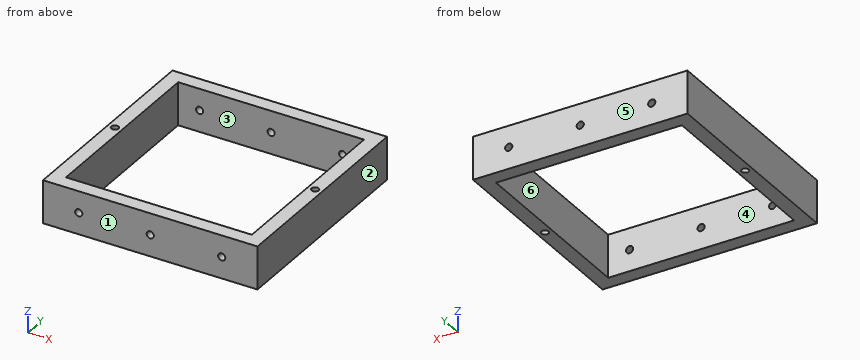
Autodesk Inventor part; units mm, degrees
ref_plane "YZ Plane" through (0, 0, 0) normal (1, 0, 0) x (0, 1, 0)
ref_plane "XZ Plane" through (0, 0, 0) normal (0, 1, 0) x (-1, 0, 0)
ref_plane "XY Plane" through (0, 0, 0) normal (0, 0, 1) x (1, 0, 0)
sketch "Boceto1" plane through (0, 0, 0) normal (0, 0, 1) x (1, 0, 0)
  line L0 (-150, 150) -> (150, 150)
  line L1 (150, 150) -> (150, -150)
  line L2 (150, -150) -> (-150, -150)
  line L3 (-150, -150) -> (-150, 150)
  line L4 (-150, 150) -> (150, -150) construction
  line L5 (150, 150) -> (-150, -150) construction
  line L6 (130, -130) -> (-130, -130)
  line L7 (-130, -130) -> (-130, 130)
  line L8 (-130, 130) -> (130, 130)
  line L9 (130, 130) -> (130, -130)
  line L10 (130, -130) -> (-130, 130) construction
  line L11 (-130, -130) -> (130, 130) construction
  point P0 (0, 0)
  dimension "d2" = 300
  dimension "d3" = 300
  dimension "d20" = 20
extrude "Extrusión1" add sketch "Boceto1" along normal blind 60
sketch "Boceto3" plane through (-150, -150, 0) normal (0, -1, 0) x (1, 0, 0)
  circle A0 centre (150, 30) radius 5
  line L0 (0, 60) -> (300, 60)
  line L1 (0, 0) -> (0, 60)
  line L2 (20, 60) -> (280, 60)
  line L3 (150, 60) -> (150, 0) construction
  circle A1 centre (250, 30) radius 5
  circle A2 centre (50, 30) radius 5
  dimension "d21" = 10
  dimension "d24" = 30
  dimension "d25" = 150
  dimension "d26" = 10
  dimension "d27" = 30
  dimension "d28" = 100
  dimension "d29" = 10
  dimension "d30" = 100
  dimension "d31" = 30
extrude "Extrusión3" cut sketch "Boceto3" against normal up to surface (300 mm away)
sketch "Boceto4" plane through (0, 0, 60) normal (0, 0, 1) x (1, 0, 0)
  circle A0 centre (-140, 0) radius 5
  line L0 (-130, -130) -> (-130, 130)
  line L1 (-150, -150) -> (150, -150)
  circle A1 centre (140, 0) radius 5
  line L2 (130, 130) -> (130, -130)
  point P0 (0, 0)
  dimension "d32" = 10
  dimension "d33" = 10
  dimension "d34" = 150
  dimension "d35" = 10
  dimension "d36" = 150
  dimension "d37" = 10
extrude "Extrusión4" cut sketch "Boceto4" against normal through all
properties part number "IdeaBase"
Read the model definition and answer for the solid it produces. Units are mm, in the model's axes. Face numbers are marked on the shaded views. A direction names the side the tool comes from. Give positions to 0.01 mm unless a question says otherwise; leave off trailing zeros. Write each loop counter-clockwise with the first axis right and the second up, starting at its lowest first coordinate (ties: lowest second). Pieces come first, ordered by that corner, then holes. Notation, with made-up numbers: (54.5, 3.25) -> (87.5, 3.25) arc R19 ccw to (87.5, 26.25) -> close; hole circle Ø10 at (65, -9). An arc over 180 degrees is marked (long way). Answer as a JSON object with one key per item and string values. Group by question number.
1) This flat-tipped pin is pushed along its axis until it touches: P1, Ø9, axis at x = -100, z = 30, coming from the -Y side. Where does it stop, or does it pass through?
2) Find section A-A (x = -100). Write down the section's boundary in (y, z).
3) Consider L1, parallel to X at y = 90, z = 16; L2, parallel to X at y = 4, z = 11. Determine where each line is inside the solid, lowest interval first. Write a range as from..to.
4) Find section B-B (y = -92.5). Write down the section's boundary in (x, z).
5) The mould has two halves that part along Y. Classify the marked faces 1, 2, 3 and 4: +Y half, -Y half, draft (parallel to the pull), parting line (faces both ways), or undercut.
6) Find section C-C (z = 47). Write down the section's boundary in (x, y).
7) A tool of negligible diameter and unlimited length cuts with its end or side. For the marked faces 5 and 6, from which of +Z, -Z, +X, -X, +Y, -Y can it reach the whole face along a straight path? Write none if from no direction.
Values follow:
{
 "1": {"P1": "passes through"},
 "2": {"outline": "(-150, 0) -> (-130, 0) -> (-130, 25) -> (-150, 25) -> close; (-150, 35) -> (-130, 35) -> (-130, 60) -> (-150, 60) -> close; (130, 0) -> (150, 0) -> (150, 25) -> (130, 25) -> close; (130, 35) -> (150, 35) -> (150, 60) -> (130, 60) -> close"},
 "3": {"L1": "x = -150..-130, 130..150", "L2": "x = -150..-143, -137..-130, 130..137, 143..150"},
 "4": {"outline": "(-150, 0) -> (-130, 0) -> (-130, 60) -> (-150, 60) -> close; (130, 0) -> (150, 0) -> (150, 60) -> (130, 60) -> close"},
 "5": {"face 1": "-Y half", "face 2": "draft", "face 3": "undercut", "face 4": "undercut"},
 "6": {"outline": "(-150, -150) -> (150, -150) -> (150, 150) -> (-150, 150) -> close; hole circle Ø10 at (-140, 0); hole (-130, -130) -> (130, -130) -> (130, 130) -> (-130, 130) -> close; hole circle Ø10 at (140, 0)"},
 "7": {"face 5": "+Z, -Z, +X, -X, +Y", "face 6": "+Z, -Z"}
}
